from build123d import *

# Parameters (mm, degrees)
F0_R            = 2.921
F1_DEPTH        = 8.001
F2_DEPTH        = 8.001
F2_COPIES_COUNT = 33
F3_SIZE         = 0.508


# Not quite as in the source:
# - a pattern or mirror of a feature is missing from the dataset's text; its kind, count and spacing are read off the source's solid


with BuildPart() as f1:
    # F0 (on Top) → F1 (new body)
    with BuildSketch(Plane.XY):
        with BuildLine():
            ThreePointArc((-0.3175, 4.8155445954), (-3.298334504, -3.5229626027), (4.826, 0))
            ThreePointArc((4.826, 0), (3.5229626027, 3.298334504), (0.3175, 4.8155445954))
            ThreePointArc((0.3175, 4.8155445954), (0, 4.826), (-0.3175, 4.8155445954))
        make_face()
        Circle(F0_R, mode=Mode.SUBTRACT)
    extrude(amount=F1_DEPTH)

    # F0 (on Top) → F2 (join, through all)
    with BuildSketch(Plane.XY):
        with BuildLine():
            ThreePointArc((-0.3175, 4.8155445954), (0, 4.826), (0.3175, 4.8155445954))
            Line((0.3175, 4.8155445954), (0.127, 5.1054))
            Line((0.127, 5.1054), (-0.127, 5.1054))
            Line((-0.127, 5.1054), (-0.3175, 4.8155445954))
        make_face()
    f2 = extrude(amount=F2_DEPTH)

    # F2_copies: F2 ×33 about axis
    f2_copies_axis = Axis((0, 0, 0), (0, 0, 1))
    for i in range(1, F2_COPIES_COUNT):
        add(f2.rotate(f2_copies_axis, i * 360 / F2_COPIES_COUNT))

    # F3
    f3_edges = [f1.edges().sort_by_distance(p)[0] for p in [
        (-2.921, 0, 8.001),
    ]]
    chamfer(f3_edges, length=F3_SIZE)


solid = f1.part
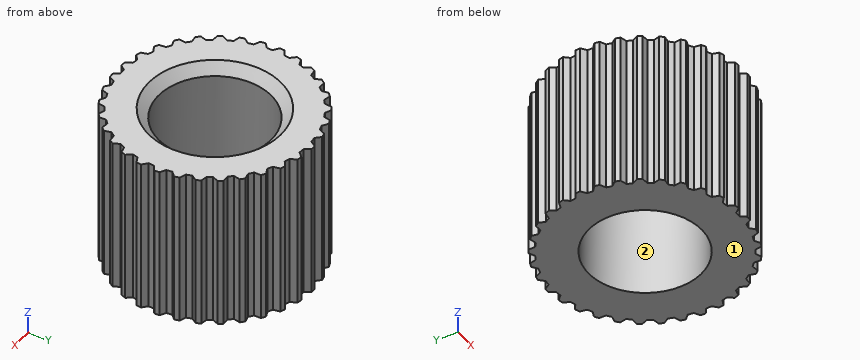
The listing builds one solid part. Answer for the finished solid, in the listing's coordinates (mm). Face numbers are marked on the shaded views. Round coordinates to 2 decimals unless told otherwise and drop trailing zeros. Use a Markdown table: item, result. Add a question column.
1. For a pull along Y with two mould halves and no side action, classify the marked faces 1 and 2 as +Y half, -Y half, draft (parallel to the pull), parting line (faces both ways), or undercut.
2. Flat-ended cylindrical pins translate along their axes: P1, Ø1, axis at y = -1.5, z = 7, coming from the -X side; P2, Ø1.5, axis at x = 2, z = 1, coming from the -Y side; P3, Ø1, axis at y = 2, z = 3, coming from the +X side. Find the tip coordinate at first contact, or state that the pin passes through.
3. Consider line 1 (Y direction, x = 0, z = 2.5); line 2 (X direction, y = -1.25, z = 7); line 3 (Y direction, x = 3, z = 5.5). Determine where each line is inside the solid, lowest interval first.
Reported:
| question | item | result |
|---|---|---|
| 1 | face 1 | draft |
| 1 | face 2 | undercut |
| 2 | P1 | x = -4.87 |
| 2 | P2 | y = -4.93 |
| 2 | P3 | x = 4.7 |
| 3 | line 1 | -4.83 to -2.92, 2.92 to 5.11 |
| 3 | line 2 | -4.66 to -2.64, 2.64 to 4.66 |
| 3 | line 3 | -4.07 to 3.78 |
